```python
from build123d import *

# Parameters (mm, degrees)
BOSS_EXTRUDE1_DEPTH = 11.4
SKETCH2_W           = 41.3
SKETCH2_H           = 11.4
BOSS_EXTRUDE2_DEPTH = 16.2
SKETCH3_R           = 5.068211815
BOSS_EXTRUDE3_DEPTH = 10


with BuildPart() as part:
    # Sketch1 → Boss-Extrude1 (new body)
    with BuildSketch(Plane.XY):
        with BuildLine():
            Line((0, 0), (-41.3, 0))
            Line((-41.3, 0), (-41.3, 13))
            Line((-41.3, 13), (-24.95603272, 13))
            Line((-24.95603272, 13), (-24.95603272, 6.95))
            ThreePointArc((-24.95603272, 6.95), (-22, 3.99396728), (-19.04396728, 6.95))
            Line((-19.04396728, 6.95), (-19.04396728, 13))
            Line((-19.04396728, 13), (-7.95603272, 13))
            Line((-7.95603272, 13), (-7.95603272, 6.95))
            ThreePointArc((-7.95603272, 6.95), (-5, 3.99396728), (-2.04396728, 6.95))
            Line((-2.04396728, 6.95), (-2.04396728, 13))
            Line((-2.04396728, 13), (0, 13))
            Line((0, 13), (0, 0))
        make_face()
    extrude(amount=BOSS_EXTRUDE1_DEPTH)

    # Sketch2 → Boss-Extrude2 (add)
    with BuildSketch(Plane.XZ):
        with Locations((-20.65, 5.7)):
            Rectangle(SKETCH2_W, SKETCH2_H)
    extrude(amount=BOSS_EXTRUDE2_DEPTH)

    # Sketch3 → Boss-Extrude3 (add)
    with BuildSketch(Plane.ZY.offset(41.3)):
        with Locations(Location((5.7, 6.192096644, 0), (0, 0, 90))):
            Circle(SKETCH3_R)
    extrude(amount=BOSS_EXTRUDE3_DEPTH)


solid = part.part
```
Could you check a few things on this model? Use its own coordinates, in mm. A direction names the side the tool comes from. Give positions to 0.01 mm unless a question says otherwise; leave off trailing zeros. Loops run counter-clockwise (first coordinate to the right, second up) from the corner with the lowest first, then second, coordinate; pieces in that order, holes last. Notation, with made-up numbers: (-12, 15.25) - (7, 15.25) arc R31 ccw to (7, 40.25) - close; hole circle Ø4 at (6.25, 26.5). An arc over 180 degrees is marked (long way). Answer in a Markdown table with one row per item. Add a question column.
Q1. For pin 1 (3.5 mm diameter, centred on y = -5, z = 5, fed in from -X), with a flat end and sliding along its axis, tell me the tip position at first contact or that it passes through.
Q2. If we section it at B-B (z = 10.25): List the corners of the cut face in (x, y) for me, plus the area to 3 significant figures.
Q3. If we section it at A-A (y = 10.25): List the corners of the cut face in (x, z) for me, plus the area to 3 significant figures.
Q4. We'd pull the mould along X, two halves only. Please class faces 4 (the face through (-19.044, 10, 6)), 5 (the face through (0, -1, 6)), 6 (the face through (-2.044, 10, 6)), 7 (the face through (-1, 13, 6)): +X half, -X half, draft (parallel to the pull), parting line (faces both ways), or undercut.
Q5. If we section it at C-C (y = -10): List the corners of the cut face in (x, z) for me.
Q6. Which directions (+Z, -Z, +X, -X, +Y, -Y) give clear straight access to the entire face, cutting with the end or side of a thin tool? Please do faces 1 (the face through (-46.23, 2.46, 2.27)), 2 (the face through (-21, -1, 11.4)), 3 (the face through (-7.956, 10, 6)).
Q7. If we section it at D-D (x = -42.5): List the corners of the cut face in (y, z) for me.
Q8. Please list where these lines run through material, in increasing order: L1, parallel to X at y = 11.5, z = 10.5; L2, parallel to X at y = 4.75, z = 8.5; L3, parallel to X at y = -0.75, z = 9. Write a range as from..to.
The answers:
| question | item | result |
|---|---|---|
| 1 | pin 1 | stops at x = -41.3 |
| 2 | outline | (-51.3, 3.96) - (-41.3, 3.96) - (-41.3, -16.2) - (0, -16.2) - (0, 13) - (-2.04, 13) - (-2.04, 6.95) arc R2.96 cw to (-7.96, 6.95) - (-7.96, 13) - (-19.04, 13) - (-19.04, 6.95) arc R2.96 cw to (-24.96, 6.95) - (-24.96, 13) - (-41.3, 13) - (-41.3, 8.42) - (-51.3, 8.42) - close |
| 2 | area | 1,150 mm^2 |
| 3 | outline | (-51.3, 2.66) - (-41.3, 2.66) - (-41.3, 0) - (-24.96, 0) - (-24.96, 11.4) - (-41.3, 11.4) - (-41.3, 8.74) - (-51.3, 8.74) - close; (-19.04, 0) - (-7.96, 0) - (-7.96, 11.4) - (-19.04, 11.4) - close; (-2.04, 0) - (0, 0) - (0, 11.4) - (-2.04, 11.4) - close |
| 3 | area | 397 mm^2 |
| 4 | face 4 | undercut |
| 4 | face 5 | +X half |
| 4 | face 6 | undercut |
| 4 | face 7 | draft |
| 5 | outline | (-41.3, 0) - (0, 0) - (0, 11.4) - (-41.3, 11.4) - close |
| 6 | face 1 | -X |
| 6 | face 2 | +Z, +X, -X, +Y, -Y |
| 6 | face 3 | +Z, -Z, +Y |
| 7 | outline | circle Ø10.14 at (6.19, 5.7) |
| 8 | L1 | x = -41.3..-24.96, -19.04..-7.96, -2.04..0 |
| 8 | L2 | x = -51.3..-23.97, -20.03..-6.97, -3.03..0 |
| 8 | L3 | x = -41.3..0 |
